Verification items for the finished model (mm, model axes). Face numbers are marked on the shaded views. Round coordinates to 2 decimals unless told otherwise and drop trailing zeros. Write each loop counter-clockwise with the first axis right and the second up, starting at its lowest first coordinate (ties: lowest second). Pieces come first, ordered by that corner, then holes.
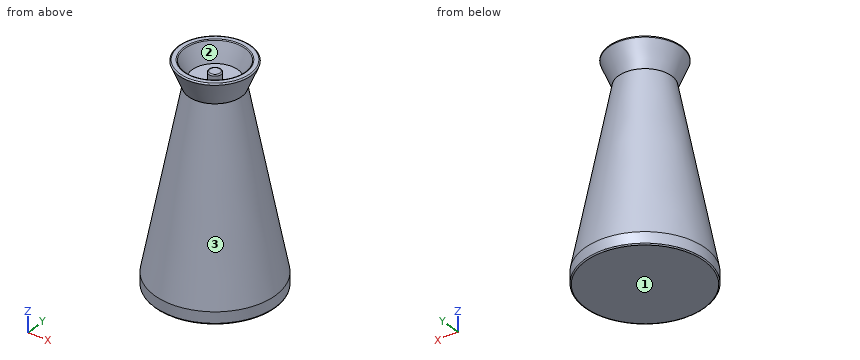
from build123d import *

# Parameters (mm, degrees)
F5_R = 5
F6_R = 5
F7_R = 5
F8_R = 5


with BuildPart() as f3:
    # F0 (on Front) → F3 (revolve)
    with BuildSketch(Plane.XZ):
        Polygon((-275.435489, 0), (0, 0), (0, 859.48139), (-120.990893, 859.48139), (-275.435489, 54.919829), align=None)
    revolve(axis=Axis((0, 0, 550.116003), (0, 0, 1)))

    # F2 (on Front) → F4 (revolve)
    with BuildSketch(Plane.XZ):
        Polygon((-168.598086, 974.709213), (-120.936424, 859.394491), (0, 859.254301), (0, 925.640881), (-28.12794, 925.640881), (-28.12794, 891.966522), (-104.616828, 891.966522), (-139.253303, 974.709213), align=None)
    revolve(axis=Axis((0, 0, 550.116003), (0, 0, 1)))

    # F5
    f5_edges = [f3.edges().sort_by_distance(p)[0] for p in [
        (168.598086, 0, 974.709213),
    ]]
    fillet(f5_edges, radius=F5_R)

    # F6
    f6_edges = [f3.edges().sort_by_distance(p)[0] for p in [
        (139.253303, 0, 974.709213),
    ]]
    fillet(f6_edges, radius=F6_R)

    # F7
    f7_edges = [f3.edges().sort_by_distance(p)[0] for p in [
        (28.12794, 0, 925.640881),
    ]]
    fillet(f7_edges, radius=F7_R)

    # F8
    f8_edges = [f3.edges().sort_by_distance(p)[0] for p in [
        (275.435489, 0, 0),
    ]]
    fillet(f8_edges, radius=F8_R)


solid = f3.part
Q1. Material ranges on line 1 along Z through (x, y) = (-69, -13.5); line 2 along Y through (x, z) = (0, 562.5); line 3 along X through (y, z) = (102, 54.5), recorded low to high.
Recorded:
line 1: z = 0 to 891.97
line 2: y = -178 to 178
line 3: x = -255.85 to 255.85
Q2. Sectioned sample at C-C (z = 361). Enter the section's corners in (x, y).
Recorded:
outline: circle Ø433.36 at (0, 0)
Q3. Sectioned sample at D-D (z = 706.5). Enter the section's corners in (x, y).
Recorded:
outline: circle Ø300.71 at (0, 0)
Q4. Depth check by flat-ended pin: P1, Ø5, axis at x = 32, z = 831, coming from the +Y side; P2, Ø5, axis at x = -149, z = 131, coming from the -Y side; P3, Ø12, axis at x = 82.5, z = 130, coming from the -Y side. Enter the tip coordinate at first touch or a pass-through.
Recorded:
P1: stops at y = 123.15
P2: stops at y = -215.9
P3: stops at y = -249.92
Q5. Release check for a two-part mould opening along Y. For the marked faces 1, 2 and 3 record: released by +Y, released by -Y, zero draft, split by the parting line, or undercut.
Recorded:
face 1: zero draft
face 2: undercut
face 3: split by the parting line
